```python
from build123d import *

# Parameters (mm, degrees)
F1_DEPTH = 1.6


with BuildPart() as f1:
    # F0 (on Top) → F1 (new body, symmetric)
    with BuildSketch(Plane.XY):
        with BuildLine():
            Line((-12.2, 3.2), (-12.2, 0))
            add(Edge.make_bspline(
                [(-12.2, 0), (-9.5769935198, -6.7725167316), (-6.9539870396, -13.5450334632), (-4.3309805594, -17.5)],
                knots=[0, 0, 0, 0, 0.3225007967, 0.3225007967, 0.3225007967, 0.3225007967], degree=3))
            Line((-4.3309805594, -17.5), (4.3309805594, -17.5))
            add(Edge.make_bspline(
                [(4.3309805594, -17.5), (6.9539870396, -13.5450334632), (9.5769935198, -6.7725167316), (12.2, 0)],
                knots=[0.6774992033, 0.6774992033, 0.6774992033, 0.6774992033, 1, 1, 1, 1], degree=3))
            Line((12.2, 0), (6.1, 0))
            Line((6.1, 0), (6.1, 3.2))
            Line((6.1, 3.2), (0, 3.2))
            Line((0, 3.2), (0, 0))
            Line((0, 0), (-6.1, 0))
            Line((-6.1, 0), (-6.1, 3.2))
            Line((-6.1, 3.2), (-12.2, 3.2))
        make_face()
    extrude(amount=F1_DEPTH, both=True)


solid = f1.part
```
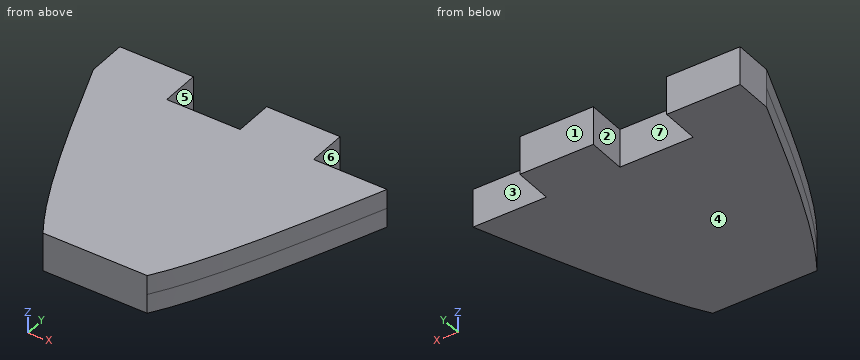
Can you work these out from the model? Positions are in its coordinate system, mm. Face numbers are marked on the shaded views. A direction names the side the tool comes from. Round coordinates to 2 decimals unless told otherwise and drop trailing zeros. Loops run counter-clockwise (first coordinate to the right, second up) from the corner with the lowest first, then second, coordinate; pieces in that order, holes last. Notation, with made-up numbers: (15.25, 82) -> (44.25, 82) arc R20 cw to (44.25, 117) -> close; hole circle Ø5 at (0, 40.5). An arc over 180 degrees is marked (long way). One line per item, written item: value. Start each with the question number.
1. If we mould it in two halves opening along X, with no side actions, what happens to the marked faces 4, 5, 6 and 7? For each: pulls with the +X half, pulls with the -X half, needs draft (parallel to the pull), parting line crosses it, or undercut.
2. For the marked faces 1, 2 and 3, which set-ups out of +Z, -Z, +X, -X, +Y, -Y let a thin tool reach every point of the face, with its end or its side?
3. For pin 1 (1 mm diameter, centred on y = -2.5, z = -0.5, fed in from +X); pin 2 (1 mm diameter, centred on x = -9.5, z = -1, fed in from -Y); pin 3 (1.6 mm diameter, centred on x = 10, z = 0, fed in from +Y), each with a flat end and sliding along its axis, tell me the tip position at first contact or that it passes through.
4. If I drill on probe 1 along X at (y, z) = (1.25, 0.7); probe 2 along Y at (x, z) = (-1.5, -1.15); probe 3 along Y at (x, z) = (-8.75, 1.2), over which ranges is the centre line in solid material (lowest first)?
5. If we section it at B-B, the plane x = -0.75: Write out the boundary of the cut face in (y, z).
6. If we section it at A-A, the plane y = 1.75: Write out the boundary of the cut face in (x, z), then the cut area to 3 significant figures.
Calculated:
1. face 4: needs draft
1. face 5: undercut
1. face 6: pulls with the +X half
1. face 7: undercut
2. face 1: +Z, -Z, +X, -X, +Y
2. face 2: +Z, -Z, +Y
2. face 3: +Z, -Z, +X, +Y
3. pin 1: stops at x = 11.42
3. pin 2: stops at y = -8.07
3. pin 3: stops at y = 0
4. probe 1: x = -12.2 to -6.1, 0 to 6.1
4. probe 2: y = -17.5 to 0
4. probe 3: y = -8.67 to 3.2
5. outline: (-17.5, -1.6) -> (0, -1.6) -> (0, 1.6) -> (-17.5, 1.6) -> close
6. outline: (-12.2, -1.6) -> (-6.1, -1.6) -> (-6.1, 1.6) -> (-12.2, 1.6) -> close; (0, -1.6) -> (6.1, -1.6) -> (6.1, 1.6) -> (0, 1.6) -> close
6. area: 39.0 mm²
